Here's the drawing with two shaded views (mm, measured from the low corner). I have some questions. A direction names the side the tool comes from. Round coordinates to 2 decimals unless told otherwise and drop trailing zeros. Loops run counter-clockwise (first coordinate to the right, second up) from the corner with the lowest first, then second, coordinate; pieces in that order, holes last. Notation, with made-up numbers: M 41.25,3.5 L 90.25,3.5 A31 cw 90.25,28.5 Z; hole C -28.75,40 d7. An arc over 180 degrees is marked long. Answer as a JSON object with one key per item and string values.
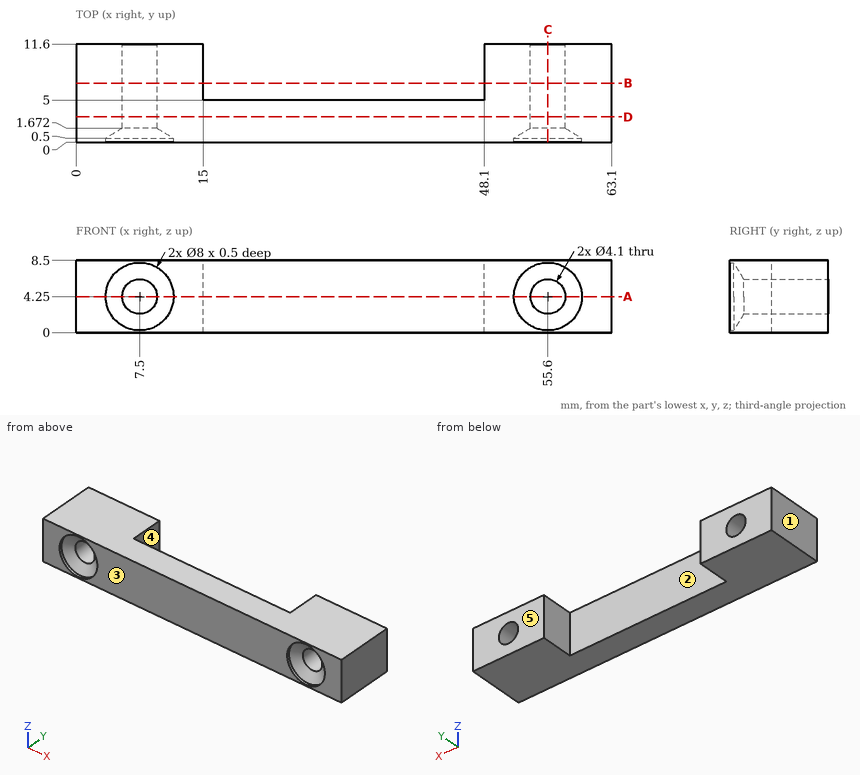
Item 1: If I drill on L1, parallel to X at y = 6, z = 4.25; L2, parallel to X at y = 0.2, z = 4.25; L3, parallel to Z at x = 7.5, y = 6, over which ranges is the centre line in solid material (lowest first)? Write a range as from..to.
Solution:
{"L1": "x = 0..5.45, 9.55..15, 48.1..53.55, 57.65..63.1", "L2": "x = 0..3.5, 11.5..51.6, 59.6..63.1", "L3": "z = 0..2.2, 6.3..8.5"}
Item 2: I want a section at D-D on y = 3. List the corners of the cut face in (x, z) for me, plus the area to 3 significant figures.
Solution:
{"outline": "M 0,0 L 63.1,0 L 63.1,8.5 L 0,8.5 Z; hole C 7.5,4.25 d4.1; hole C 55.6,4.25 d4.1", "area": "510 mm2"}
Item 3: I want a section at C-C on x = 55.6. List the corners of the cut face in (y, z) for me.
Solution:
{"outline": "M 0,0 L 11.6,0 L 11.6,2.2 L 1.67,2.2 L 0.5,0.25 L 0,0.25 Z; M 0,8.25 L 0.5,8.25 L 1.67,6.3 L 11.6,6.3 L 11.6,8.5 L 0,8.5 Z"}
Item 4: For P1, Ø2.5, axis at x = 55.6, z = 4.25, coming from the -Y side; P2, Ø4, axis at x = 27.5, z = 4.5, coming from the +Y side; P3, Ø4, axis at x = 6.5, z = 3, coming from the -Y side, each with a flat end and sliding along its axis, tell me the tip position at first contact or that it passes through.
Solution:
{"P1": "passes through", "P2": "stops at y = 5", "P3": "stops at y = 0.74"}
Item 5: For the marked faces 4 and 5, which set-ups out of +Z, -Z, +X, -X, +Y, -Y let a thin tool reach every point of the face, with its end or its side?
Solution:
{"face 4": "+Z, -Z, +Y", "face 5": "+Z, -Z, +X, -X, +Y"}
Item 6: I want a section at B-B on y = 7. List the corners of the cut face in (x, z) for me.
Solution:
{"outline": "M 0,0 L 15,0 L 15,8.5 L 0,8.5 Z; M 48.1,0 L 63.1,0 L 63.1,8.5 L 48.1,8.5 Z; hole C 7.5,4.25 d4.1; hole C 55.6,4.25 d4.1"}
Item 7: We'd pull the mould along X, two halves only. Please class the marked faces 1, 2 and 3: +X half, -X half, draft (parallel to the pull), parting line (faces both ways), or undercut.
Solution:
{"face 1": "-X half", "face 2": "undercut", "face 3": "draft"}
Item 8: I want a section at A-A on z = 4.25. List the corners of the cut face in (x, y) for me.
Solution:
{"outline": "M 0,0 L 3.5,0 L 3.5,0.5 L 5.45,1.67 L 5.45,11.6 L 0,11.6 Z; M 9.55,1.67 L 11.5,0.5 L 11.5,0 L 51.6,0 L 51.6,0.5 L 53.55,1.67 L 53.55,11.6 L 48.1,11.6 L 48.1,5 L 15,5 L 15,11.6 L 9.55,11.6 Z; M 57.65,1.67 L 59.6,0.5 L 59.6,0 L 63.1,0 L 63.1,11.6 L 57.65,11.6 Z"}
